Geometry check sheet. Reference: the model listing, model coordinates, mm. A direction names the side the tool comes from. Coordinates: 2 decimals unless noted, no trailing zeros. Loops run counter-clockwise (first coordinate to the right, second up) from the corner with the lowest first, then second, coordinate; pieces in that order, holes last.
from build123d import *

# Parameters (mm, degrees)
SKETCH2_R           = 9.25
SKETCH2_R_2         = 4
BOSS_EXTRUDE1_DEPTH = 4.8
HOLE1_D             = 1.9
HOLE1_DEPTH         = 4.801
HOLE1_CBORE_D       = 2.35
HOLE1_CBORE_DEPTH   = 1
CIRPATTERN1_COUNT   = 13


with BuildPart() as part:
    # Sketch2 → Boss-Extrude1 (new body)
    with BuildSketch(Plane(origin=(0, 0, 0), x_dir=(1, 0, 0), z_dir=(0, 1, 0))):
        Circle(SKETCH2_R)
        Circle(SKETCH2_R_2, mode=Mode.SUBTRACT)
    extrude(amount=BOSS_EXTRUDE1_DEPTH)

    # Hole1
    with Locations(Plane(origin=(0, 4.8, 0), x_dir=(1, 0, 0), z_dir=(0, 1, 0))):
        with Locations((0, 5.5)):
            hole1 = CounterBoreHole(HOLE1_D / 2, HOLE1_CBORE_D / 2, HOLE1_CBORE_DEPTH, depth=HOLE1_DEPTH)

    # CirPattern1: Hole1 ×13 about axis
    cirpattern1_axis = Axis((0, 0, 0), (0, 1, 0))
    for i in range(1, CIRPATTERN1_COUNT):
        add(hole1.rotate(cirpattern1_axis, i * 360 / CIRPATTERN1_COUNT), mode=Mode.SUBTRACT)


solid = part.part
1) Access from +Z, -Z, +X, -X, +Y, -Y to the whole of each face (thin tool, end or side, straight path). Record for faces 3 (the cylindrical face through (3.416, 1.873, -4.466)), 4 (the cylindrical face through (-0.25, 4.31, -4.35)).
Data:
face 3: +Y, -Y
face 4: +Y
2) Section check C-C on x = 7.5. Record the cut outline in (y, z), and give its area (3 significant figures).
Data:
outline: (0, -5.41) - (4.8, -5.41) - (4.8, 5.41) - (0, 5.41) - close
area: 52.0 mm2
3) Material ranges on probe 1 along Z at (x, y) = (-5.25, 3.5); probe 2 along Z at (x, y) = (-1, 2.25); probe 3 along X at (y, z) = (4.2, -5.5) (3 decimals), recorded low to high.
Data:
probe 1: z = -7.62 to -3.74, -2.51 to -1.59, 0.26 to 1.01, 2.89 to 7.62
probe 2: z = -9.2 to -3.87, 3.87 to 4.44, 6.24 to 9.2
probe 3: x = -7.437 to -3.548, -1.564 to -1.175, 1.175 to 1.564, 3.548 to 7.437
4) Depth check by flat-ended pin: pin 1 (1.5 mm diameter, centred on x = 3.5, y = 3.5, fed in from +Z); pin 2 (1.2 mm diameter, centred on x = -3.5, z = 4.5, fed in from +Y); pin 3 (1 mm diameter, centred on x = 4, y = 3, fed in from -Z). Enter the tip coordinate at first touch or a pass-through.
Data:
pin 1: stops at z = 8.83
pin 2: stops at y = 3.8
pin 3: stops at z = -8.56
5) Section check A-A on z = 0. Record the cut outline in (x, y), and give its area (3 significant figures).
Data:
outline: (-9.25, 0) - (-6.14, 0) - (-6.14, 3.8) - (-6.43, 3.8) - (-6.43, 4.8) - (-9.25, 4.8) - close; (-4.78, 0) - (-4, 0) - (-4, 4.8) - (-4.49, 4.8) - (-4.49, 3.8) - (-4.78, 3.8) - close; (4, 0) - (4.78, 0) - (4.78, 3.8) - (4.49, 3.8) - (4.49, 4.8) - (4, 4.8) - close; (6.14, 0) - (9.25, 0) - (9.25, 4.8) - (6.43, 4.8) - (6.43, 3.8) - (6.14, 3.8) - close
area: 36.2 mm2
6) Section check D-D on z = 7.5. Record the cut outline in (x, y).
Data:
outline: (-5.41, 0) - (5.41, 0) - (5.41, 4.8) - (-5.41, 4.8) - close
7) Section check B-B on y = 0.9. Count the separate pieces of the cut face and the enclosed holes in it, and give its area (3 significant figures).
Data:
separate pieces: 1
enclosed holes: 14
area: 182 mm2
8) Mould release check, pull along X, two halves, no side actions. Record for faces 1 (the flat face through (-4.2, 0, -0.1)), 2 (the cylindrical face through (-4.777, 4.307, 4.44)): +X half, -X half, draft (parallel to the pull), parting line (faces both ways), or undercut.
Data:
face 1: draft
face 2: undercut
